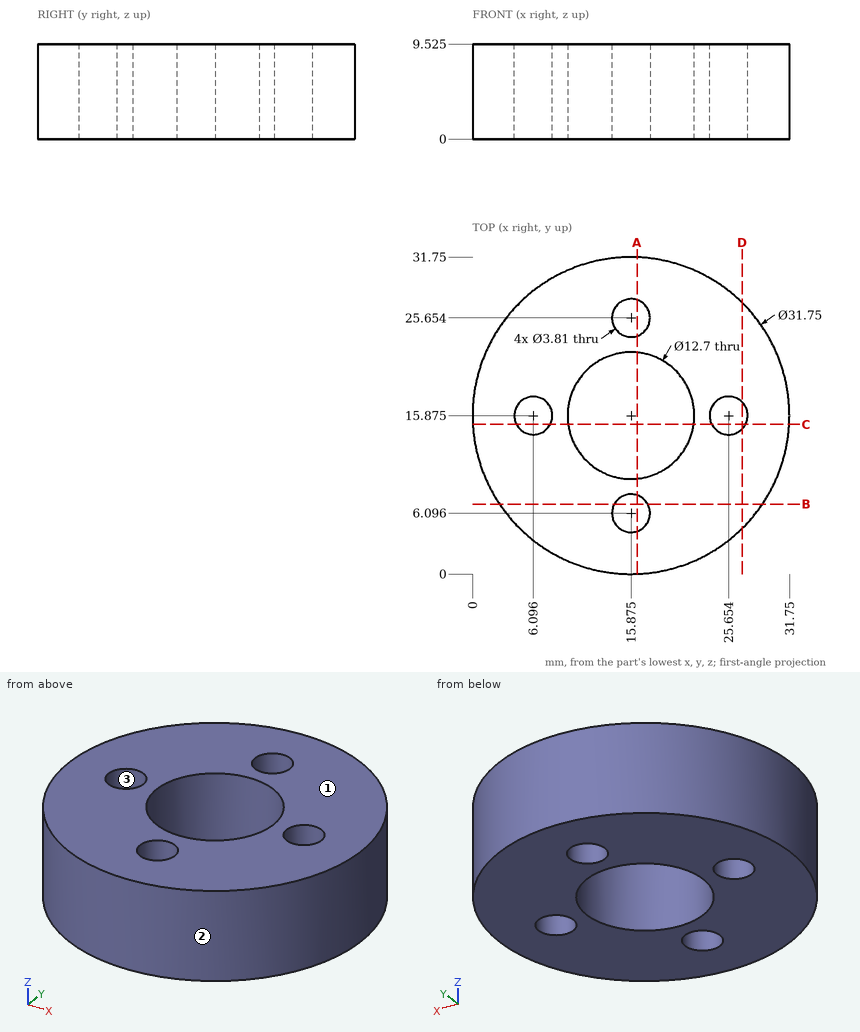
Job drawing, mm, ordinate dimensions from the low corner. One solid piece. Give positions to 0.01 mm unless a question says otherwise; leave off trailing zeros. Write each loop counter-clockwise with the first axis right and the second up, starting at its lowest first coordinate (ties: lowest second). Pieces come first, ordered by that corner, then holes. Notation, with made-up numbers: (-27, 87) - (9, 87) arc R23 ccw to (9, 118) - close; hole circle Ø7 at (0, 23.5). An arc over 180 degrees is marked (long way). Answer as CSV lines item,"result".
1. Band-saw the part on B-B (y = 7). Write the cut outline in (x, z) (3 decimals).
Responses:
outline,"(2.713, 0) - (14.198, 0) - (14.198, 9.525) - (2.713, 9.525) - close; (17.552, 0) - (29.037, 0) - (29.037, 9.525) - (17.552, 9.525) - close"
2. Pin check, flat tips, straight feed: pin 1 (4.5 mm diameter, centred on x = 15.875, y = 25.654, fed in from -Z); pin 2 (4 mm diameter, centred on x = 13, z = 3, fed in from +Y); pin 3 (4 mm diameter, centred on x = 5.5, z = 2.5, fed in from +Y); pin 4 (5 mm diameter, centred on x = 13, z = 2, fed in from -Y). Stop position of each tip, or through.
Responses:
pin 1,"stops at z = 0"
pin 2,"stops at y = 31.73"
pin 3,"stops at y = 29.36"
pin 4,"stops at y = 0"
3. Drill centre lines: L1, parallel to Y at x = 16, z = 1.25; L2, parallel to Y at x = 17.5, z = 2; L3, parallel to X at y = 19, z = 8.5. Where is each one in solid material? Low to high. Write a range as [from, to].
Responses:
L1,"y = [0, 4.2], [8, 9.53], [22.22, 23.75], [27.55, 31.75]"
L2,"y = [0.08, 5.1], [7.09, 9.74], [22.01, 24.66], [26.65, 31.67]"
L3,"x = [0.31, 10.35], [21.4, 31.44]"
4. Band-saw the part on D-D (x = 27). Write the cut outline in (y, z) (3 decimals), and give its area (3 significant figures).
Responses:
outline,"(4.55, 0) - (14.527, 0) - (14.527, 9.525) - (4.55, 9.525) - close; (17.223, 0) - (27.2, 0) - (27.2, 9.525) - (17.223, 9.525) - close"
area,"190 mm2"
5. Band-saw the part on C-C (y = 15). Write the cut outline in (x, z) (3 decimals).
Responses:
outline,"(0.024, 0) - (4.404, 0) - (4.404, 9.525) - (0.024, 9.525) - close; (7.788, 0) - (9.586, 0) - (9.586, 9.525) - (7.788, 9.525) - close; (22.164, 0) - (23.962, 0) - (23.962, 9.525) - (22.164, 9.525) - close; (27.346, 0) - (31.726, 0) - (31.726, 9.525) - (27.346, 9.525) - close"
6. Band-saw the part on A-A (x = 16.5). Write the cut outline in (y, z) (3 decimals).
Responses:
outline,"(0.012, 0) - (4.296, 0) - (4.296, 9.525) - (0.012, 9.525) - close; (7.896, 0) - (9.556, 0) - (9.556, 9.525) - (7.896, 9.525) - close; (22.194, 0) - (23.854, 0) - (23.854, 9.525) - (22.194, 9.525) - close; (27.454, 0) - (31.738, 0) - (31.738, 9.525) - (27.454, 9.525) - close"
7. Two-plate mould, pull along X, no slides. Class the marked faces 1, 2 and 3: +X half, -X half, draft (parallel to the pull), parting line (faces both ways), or undercut.
Responses:
face 1,"draft"
face 2,"parting line"
face 3,"undercut"
